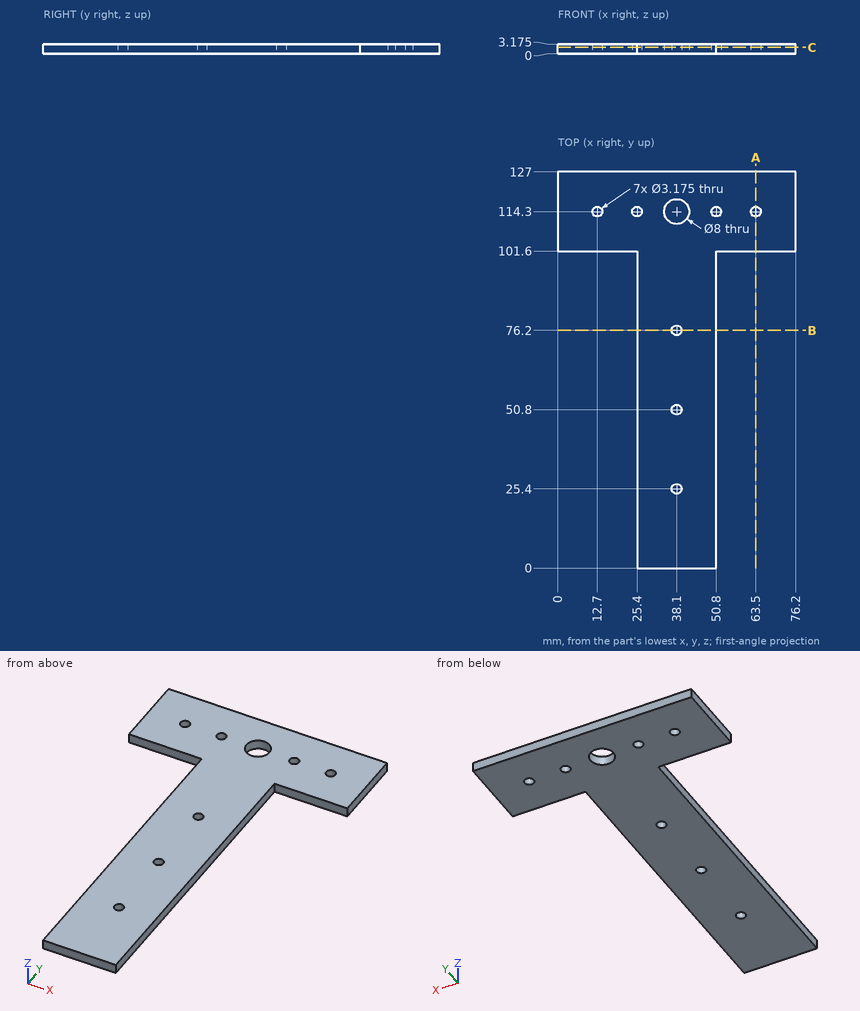
Geometry: see drawing. Coordinates: mm, zero at the bounding-box minimum. Give positions to 0.01 mm unless a question says otherwise; leave off trailing zeros. Loops run counter-clockwise (first coordinate to the right, second up) from the corner with the lowest first, then second, coordinate; pieces in that order, holes last. Notation, with made-up numbers: (29.5, 81.5) - (58.5, 81.5) arc R11 cw to (58.5, 101.5) - close; hole circle Ø1 at (79.25, -19). An arc over 180 degrees is marked (long way). Use CSV: the item, a comma, the result in double quotes. Start each with the question number.
1. Pin query (flat end, axial travel): pin 1 (1 mm diameter, centred on x = 69.5, z = 1, fed in from -Y); pin 2 (5 mm diameter, centred on x = 12.7, y = 114.3, fed in from -Z); pin 3 (1.6 mm diameter, centred on y = 61.5, z = 1, fed in from +X). Return the tip coordinate at first contact, or that it passes through.
2. Section B-B (y = 76.2). Output: boundary loops of the cut face in (x, z) (1 decimal), then the cut area to 3 significant figures.
3. Section C-C (z = 2.1). Count the separate pieces of the cut face and the enclosed holes in it, then the cut area to 3 significant figures.
4. Section A-A (x = 63.5). Output: boundary loops of the cut face in (y, z) (1 decimal).
5. Ray query, L1, parallel to Y at x = 38.1, z = 0.95; L2, parallel to X at y = 76.2, z = 2.3; L3, parallel to Y at x = 63.5, z = 2.05. Return the intervals inside material, ascending.
Response:
1,pin 1,"y = 101.6"
1,pin 2,"z = 0"
1,pin 3,"x = 50.8"
2,outline,"(25.4, 0) - (36.5, 0) - (36.5, 3.2) - (25.4, 3.2) - close; (39.7, 0) - (50.8, 0) - (50.8, 3.2) - (39.7, 3.2) - close"
2,area,"70.6 mm²"
3,separate pieces,"1"
3,enclosed holes,"8"
3,area,"4,410 mm²"
4,outline,"(101.6, 0) - (112.7, 0) - (112.7, 3.2) - (101.6, 3.2) - close; (115.9, 0) - (127, 0) - (127, 3.2) - (115.9, 3.2) - close"
5,L1,"0 to 23.81, 26.99 to 49.21, 52.39 to 74.61, 77.79 to 110.3, 118.3 to 127"
5,L2,"25.4 to 36.51, 39.69 to 50.8"
5,L3,"101.6 to 112.71, 115.89 to 127"
